The listing builds one solid part. Answer for the finished solid, in the listing's coordinates (mm). Face numbers are marked on the shaded views. A direction names the side the tool comes from. Give positions to 0.01 mm unless a question says otherwise; leave off trailing zeros. Write each loop counter-clockwise with the first axis right and the second up, starting at its lowest first coordinate (ties: lowest second). Pieces come first, ordered by that corner, then holes. Notation, with made-up numbers: M 7.25,3 L 64.25,3 A31 cw 64.25,42 Z; hole C 60,42.25 d10. An arc over 180 degrees is marked long. Answer as a JSON object with one key per item and string values.
Autodesk Inventor part; units mm, degrees
ref_plane "YZ Plane" through (0, 0, 0) normal (1, 0, 0) x (0, 1, 0)
ref_plane "XZ Plane" through (0, 0, 0) normal (0, 1, 0) x (-1, 0, 0)
ref_plane "XY Plane" through (0, 0, 0) normal (0, 0, 1) x (1, 0, 0)
sketch "Sketch1" plane through (0, 0, 0) normal (0, 0, 1) x (1, 0, 0)
  circle A0 centre (6.35, 64.0658) radius 6.35
  circle A1 centre (58.0536, 32.9878) radius 6.35
  line L0 (0, 0) -> (33.7266, 0)
  circle A2 centre (50.6167, 92.4839) radius 2.7589
  circle A3 centre (52.5819, 79.7839) radius 2.7589
  line L1 (0, 0) -> (0, 86.6758) construction
  dimension "d12" = 12.7
  dimension "d13" = 12.7
  dimension "d15" = 51.7036
  dimension "d16" = 31.078
  dimension "d18" = 32.9877
  dimension "d19" = 24.327
  dimension "d20" = 5.5178
  dimension "d21" = 5.5178
  dimension "d22" = 46.7962
  dimension "d23" = 5.4717
  dimension "d24" = 1.9652
  dimension "d25" = 12.7
sketch "Sketch3" plane through (0, 0, 0) normal (0, 0, 1) x (1, 0, 0)
  circle A0 centre (6.35, 64.0658) radius 6.35
  circle A1 centre (50.6167, 92.4839) radius 2.7589
  circle A2 centre (52.5819, 79.7839) radius 2.7589
  circle A3 centre (58.0536, 32.9878) radius 6.35
  circle A4 centre (6.35, 64.0658) radius 9.525
  circle A5 centre (58.0536, 32.9878) radius 9.525
  circle A6 centre (52.5819, 79.7839) radius 5.9339
  circle A7 centre (50.6167, 92.4839) radius 5.9339
  line L0 (0, 0) -> (-3.1632, 63.5926)
  line L1 (33.7266, 0) -> (64.1959, 25.7078)
  line L2 (1.7635, 72.4138) -> (47.7594, 97.6846)
  line L3 (56.4808, 93.3913) -> (58.446, 80.6913)
  line L4 (58.406, 80.9203) -> (67.4023, 34.8118)
  line L5 (6.35, 64.0658) -> (58.0536, 32.9878) construction
  line L6 (58.0536, 32.9878) -> (52.5819, 79.7839) construction
  line L7 (52.5819, 79.7839) -> (50.6167, 92.4839) construction
  line L8 (50.6167, 92.4839) -> (6.35, 64.0658) construction
  line L9 (52.5819, 79.7839) -> (6.35, 64.0658) construction
  line L10 (0, 0) -> (33.7266, 0)
  line L11 (0, 0) -> (33.7266, 0)
  line L12 (33.7266, 0) -> (33.7266, -31.75)
  line L13 (33.7266, -31.75) -> (0, -31.75)
  line L14 (0, -31.75) -> (0, 0)
  point P0 (58.4282, 80.8062)
  dimension "d27" = 3.175
  dimension "d28" = 3.175
  dimension "d29" = 3.175
  dimension "d30" = 3.175
  dimension "d33" = 31.75
extrude "Plate3" add sketch "Sketch3" along normal blind 3.048 contours A4 | A6 | A4 L2 A7 L3 L4 A5 L1 L10 L0 | A7 | A5
sketch "Sketch4" plane through (0, -3.048, -3.048) normal (0, -1, 0) x (1, 0, 0)
  line L0 (33.7266, 0) -> (0, 0)
  line L1 (0, 0) -> (0, -25.654)
  line L2 (0, -25.654) -> (33.7266, -25.654)
  line L3 (33.7266, -25.654) -> (33.7266, 0)
edge flange "Flange1" height 31.75 angle 90 thickness 3.048 bend radius 3.048 thickness toward (0, -1, 0) relief tear relief width 3.048 relief depth 1.524 edges at (16.8633, 0, 0) wall of the first edge with corners at (33.7266, -3.048, -3.048) (0, -3.048, -3.048) (0, -3.048, -28.702) (33.7266, -3.048, -28.702)
bend "Bend3"
corner "Corner1"
equation "\"d21\" = d20"
equation "\"d28\" = d27"
equation "\"d29\" = d27"
equation "\"d30\" = d27"
equation "\"d31\" = Thickness"
equation "\"d34\" = BendReliefWidth"
equation "\"d35\" = BendReliefDepth"
equation "\"d36\" = MinimumRemnant"
equation "\"d37\" = TransitionRadius"
equation "\"d40\" = BendRadius"
equation "\"d41\" = CornerReliefSize"
equation "\"d42\" = GapSize"
equation "\"d43\" = JacobiRadiusSize"
equation "\"BendRadius\" = Thickness"
equation "\"BendReliefWidth\" = Thickness"
equation "\"BendReliefDepth\" = 0.5 * Thickness"
equation "\"CornerReliefSize\" = 4 * Thickness"
equation "\"MinimumRemnant\" = 2 * Thickness"
equation "\"TransitionRadius\" = BendRadius"
equation "\"JacobiRadiusSize\" = BendRadius"
equation "\"GapSize\" = Thickness"
properties part number "GearsMount"
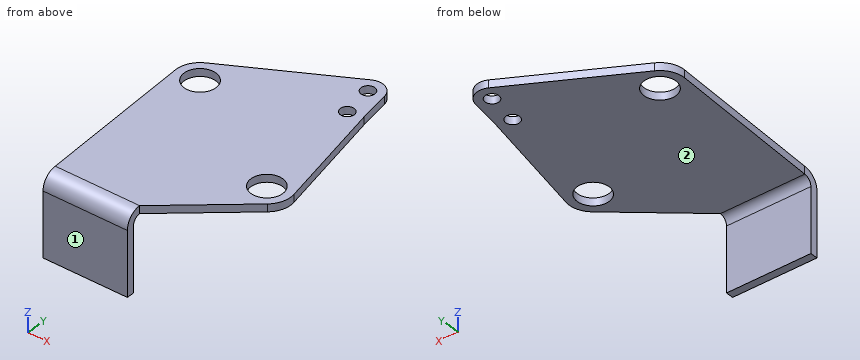
1. Flat-ended cylindrical pins translate along their axes: pin 1 (5 mm diameter, centred on y = -2, z = -16.5, fed in from -X); pin 2 (10 mm diameter, centred on x = 58.05, y = 32.99, fed in from +Z); pin 3 (5 mm diameter, centred on y = -1.5, z = -10, fed in from +X); pin 4 (8 mm diameter, centred on x = 59.5, y = 37.5, fed in from -Z). Find the tip coordinate at first contact, or state that the pin passes through.
Verdict:
{"pin 1": "stops at x = 0", "pin 2": "passes through", "pin 3": "stops at x = 33.73", "pin 4": "stops at z = 0"}
2. Consider line 1 along Y through (x, z) = (16, -20); line 2 along Z through (x, y) = (57.5, 63.5); line 3 along X through (y, z) = (87, 1.5). Determine where each line is inside the solid, lowest interval first.
Verdict:
{"line 1": "y = -6.1 to -3.05", "line 2": "z = 0 to 3.05", "line 3": "x = 28.31 to 57.47"}
3. A cutting plane is placed at B-B, the plane x = 3. Give the vertices of the cut face in (y, z).
Verdict:
{"outline": "M -6.1,-28.7 L -3.05,-28.7 L -3.05,-3.05 A3.05 cw 0,0 L 58.67,0 L 58.67,3.05 L 0,3.05 A6.1 ccw -6.1,-3.05 Z; M 69.46,0 L 73.09,0 L 73.09,3.05 L 69.46,3.05 Z"}
4. A cutting plane is placed at A-A, the plane y = 69. Give the vertices of the cut face in (x, z).
Verdict:
{"outline": "M -1.8,0 L 2.35,0 L 2.35,3.05 L -1.8,3.05 Z; M 10.35,0 L 60.73,0 L 60.73,3.05 L 10.35,3.05 Z"}
5. A cutting plane is placed at D-D, the plane z = -11. Give the vertices of the cut face in (x, y), plus the area to 3 significant figures.
Verdict:
{"outline": "M 0,-6.1 L 33.73,-6.1 L 33.73,-3.05 L 0,-3.05 Z", "area": "103 mm2"}
6. For the marked faces 1 and 2, determine the directions among +Z, -Z, +X, -X, +Y, -Y from which every point of the face is accessible in a straight line to the end or side of a thin tool.
Verdict:
{"face 1": "+Z, -Z, +X, -X, -Y", "face 2": "-Z, +X, -X, +Y"}
7. A cutting plane is placed at C-C, the plane x = 25.5. Give the vertices of the cut face in (y, z), plus the area to 3 significant figures.
Verdict:
{"outline": "M -6.1,-28.7 L -3.05,-28.7 L -3.05,-3.05 A3.05 cw 0,0 L 85.45,0 L 85.45,3.05 L 0,3.05 A6.1 ccw -6.1,-3.05 Z", "area": "361 mm2"}
